Geometry check sheet. Reference: drawing and pictorial views, mm from the part's lowest x, y, z. Give positions to 0.01 mm unless a question says otherwise; leave off trailing zeros. Loops run counter-clockwise (first coordinate to the right, second up) from the corner with the lowest first, then second, coordinate; pieces in that order, holes last. Notation, with made-up numbers: (79, 57.25) -> (101, 57.25) arc R15 ccw to (101, 81.25) -> close; hole circle Ø10 at (77, -22.75). An arc over 180 degrees is marked (long way). Write item = value, one per line. Start each with the question number.
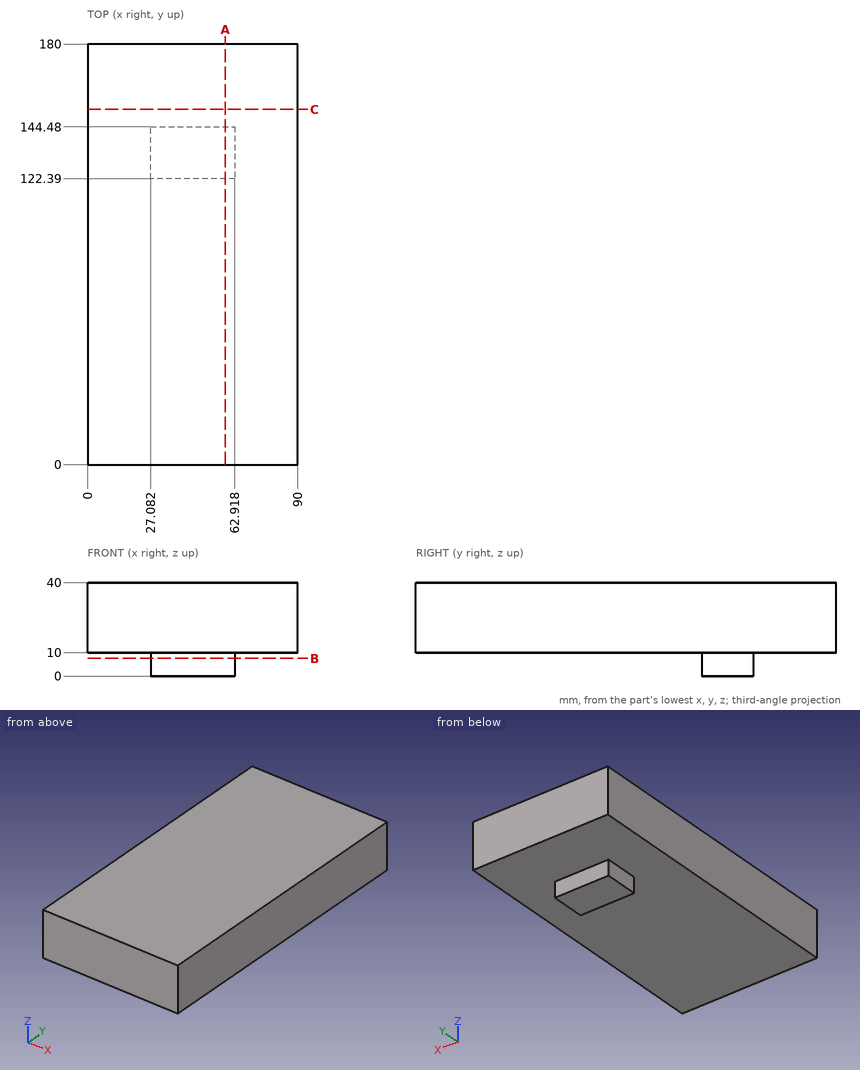
1) Thickness scan on line 1 (Z direction, x = 31, y = 84). Record the ranges inside material, lowest first.
2) Section check C-C (y = 152). Enter the section's corners in (x, z), plus the area to 3 significant figures.
3) Section check A-A (x = 59). Enter the section's corners in (y, z).
4) Section check B-B (z = 7.5). Enter the section's corners in (x, y), plus the area to 3 significant figures.
5) Depth check by flat-ended pin: pin 1 Ø3 at (x, z) = (40.5, 3) entering from +Y; pin 2 Ø8 at (x, z) = (43, 4) entering from -Y; pin 3 Ø3 at (y, z) = (135.5, 4.5) entering from -X. Enter the tip coordinate at first touch or a pass-through.
Check result:
q1.line_1 = 10 to 40
q2.outline = (0, 10) -> (90, 10) -> (90, 40) -> (0, 40) -> close
q2.area = 2,700 mm2
q3.outline = (0, 10) -> (122.39, 10) -> (122.39, 0) -> (144.48, 0) -> (144.48, 10) -> (180, 10) -> (180, 40) -> (0, 40) -> close
q4.outline = (27.08, 122.39) -> (62.92, 122.39) -> (62.92, 144.48) -> (27.08, 144.48) -> close
q4.area = 792 mm2
q5.pin_1 = 144.48
q5.pin_2 = 122.39
q5.pin_3 = 27.08
